Autodesk Inventor part; units mm, degrees
ref_plane "YZ Plane" through (0, 0, 0) normal (1, 0, 0) x (0, 1, 0)
ref_plane "XZ Plane" through (0, 0, 0) normal (0, 1, 0) x (-1, 0, 0)
ref_plane "XY Plane" through (0, 0, 0) normal (0, 0, 1) x (1, 0, 0)
sketch "Sketch1" plane through (0, 0, 0) normal (0, 1, 0) x (-1, 0, 0)
  circle A0 centre (0, 0) radius 1.8415
  circle A1 centre (0, 0) radius 2.3813
  circle A2 centre (0, -6.35) radius 1.651
  circle A3 centre (0, 6.35) radius 1.651
  arc A4 (3.4219, 7.0485) -> (-3.4219, 7.0485) centre (0, 6.35) ccw
  arc A5 (-3.4219, -7.0485) -> (3.4219, -7.0485) centre (0, -6.35) ccw
  line L0 (3.4219, 7.0485) -> (4.6663, 0.9525)
  line L1 (-3.4219, 7.0485) -> (-4.6663, 0.9525)
  line L2 (3.4219, -7.0485) -> (4.6663, -0.9525)
  line L3 (-3.4219, -7.0485) -> (-4.6663, -0.9525)
  arc A6 (4.6663, -0.9525) -> (4.6663, 0.9525) centre (0, 0) ccw
  arc A7 (-4.6663, 0.9525) -> (-4.6663, -0.9525) centre (0, 0) ccw
  dimension "d0" = 3.683
  dimension "d1" = 4.7625
  dimension "d3" = 3.302
  dimension "d4" = 3.302
  dimension "d5" = 6.985
  dimension "d6" = 6.985
  dimension "d7" = 6.35
  dimension "d8" = 6.35
  dimension "d9" = 4.7625
extrude "Extrusion1" add sketch "Sketch1" along normal blind 2.159 contours A1 | L0 A6 L2 A5 L3 A7 L1 A4
extrude "Extrusion2" add sketch "Sketch1" along normal blind 2.794 contours A1
sketch "Sketch3" plane through (0, 2.159, 0) normal (0, 1, 0) x (1, 0, 0)
  circle A0 centre (0, 0) radius 4.191
  circle A1 centre (0, 0) radius 2.3813
  dimension "d14" = 8.382
extrude "Extrusion3" cut sketch "Sketch3" against normal blind 1.27
properties part number "tetherSeal"
CAD build for the part. Positions are in the model's coordinates, mm. A direction names the side the tool comes from. Round coordinates to 2 decimals unless told otherwise and drop trailing zeros. Write each loop counter-clockwise with the first axis right and the second up, starting at its lowest first coordinate (ties: lowest second). Pieces come first, ordered by that corner, then holes. Notation, with made-up numbers: M -1.75,40.5 L 22.25,40.5 A9 ccw 22.25,50.5 Z; hole C 14,39.5 d1. An arc over 180 degrees is marked long. Use a Markdown table: item, result. Add a question column.
1. Slice it at D-D on y = 0.3. Give the cut face in (x, z).
2. 3-axis set-ups, long thin cutter, end or side, ignore diameter. For faces 4 (the face through (3.997, 1.533, -1.259)), 5 (the face through (-0.85, 1.377, 1.634)): which of +Z, -Z, +X, -X, +Y, -Y reach the whole face in a straight line?
3. Drill centre lines: probe 1 along X at (y, z) = (1.95, 1); probe 2 along Z at (x, y) = (0.25, 0.2); probe 3 along Y at (x, z) = (-2.5, 7.25). Where is each one in solid material? Low to high.
4. Slice it at B-B on z = 0. Give the cut face in (x, y).
5. Pull direction Z, two halves, no side cores. Call faces 1 (the face through (2, 0.889, 2)), 2 (the face through (-2, 0, 0)), 3 (the face through (0.07, 1.06, 9.84)): released by +Z, released by -Z, zero draft, split by the parting line, or undercut.
6. Slice it at A-A on y = 1.4. Give the cut face in (x, z), then the cut area to 3 significant figures.
7. Slice it at C-C on x = 0. Give the cut face in (y, z).
Reply:
| question | item | result |
|---|---|---|
| 1 | outline | M -4.67,-0.95 L -3.42,-7.05 A3.49 ccw 3.42,-7.05 L 4.67,-0.95 A4.76 ccw 4.67,0.95 L 3.42,7.05 A3.49 ccw -3.42,7.05 L -4.67,0.95 A4.76 ccw Z; hole C 0,0 d3.68; hole C 0,-6.35 d3.3; hole C 0,6.35 d3.3 |
| 2 | face 4 | +Y |
| 2 | face 5 | +Y, -Y |
| 3 | probe 1 | x = -4.66 to -4.07, -2.16 to -1.55, 1.55 to 2.16, 4.07 to 4.66 |
| 3 | probe 2 | z = -9.83 to -7.98, -4.72 to -1.82, 1.82 to 4.72, 7.98 to 9.83 |
| 3 | probe 3 | y = 0 to 2.16 |
| 4 | outline | M -4.76,0 L -1.84,0 L -1.84,2.79 L -2.38,2.79 L -2.38,0.89 L -4.19,0.89 L -4.19,2.16 L -4.76,2.16 Z; M 1.84,0 L 4.76,0 L 4.76,2.16 L 4.19,2.16 L 4.19,0.89 L 2.38,0.89 L 2.38,2.79 L 1.84,2.79 Z |
| 5 | face 1 | undercut |
| 5 | face 2 | zero draft |
| 5 | face 3 | released by +Z |
| 6 | outline | M -4.67,-0.95 L -3.42,-7.05 A3.49 ccw 3.42,-7.05 L 4.67,-0.95 A4.76 ccw 4.67,0.95 L 3.42,7.05 A3.49 ccw -3.42,7.05 L -4.67,0.95 A4.76 ccw Z; C 0,0 d4.76; hole C 0,0 d8.38; hole C 0,0 d3.68; hole C 0,-6.35 d3.3; hole C 0,6.35 d3.3 |
| 6 | area | 80.1 mm^2 |
| 7 | outline | M 0,-9.84 L 2.16,-9.84 L 2.16,-8 L 0,-8 Z; M 0,-4.7 L 2.16,-4.7 L 2.16,-4.19 L 0.89,-4.19 L 0.89,-2.38 L 2.79,-2.38 L 2.79,-1.84 L 0,-1.84 Z; M 0,1.84 L 2.79,1.84 L 2.79,2.38 L 0.89,2.38 L 0.89,4.19 L 2.16,4.19 L 2.16,4.7 L 0,4.7 Z; M 0,8 L 2.16,8 L 2.16,9.84 L 0,9.84 Z |
